Read the model definition and answer for the solid it produces. Units are mm, in the model's axes. Face numbers are marked on the shaded views. Round coordinates to 2 decimals unless told otherwise and drop trailing zeros. Order: outer loops, then holes, each group sorted by start corner. A loop starts at its lowest first (then second) coordinate and runs counter-clockwise, first axis right, second up. Notation, with made-up numbers: M 57.25,-31 L 92.25,-31 A24 ccw 92.25,-16 Z; hole C -2.75,11 d3. An arc over 180 degrees is marked long. Answer as CSV lines item,"result".
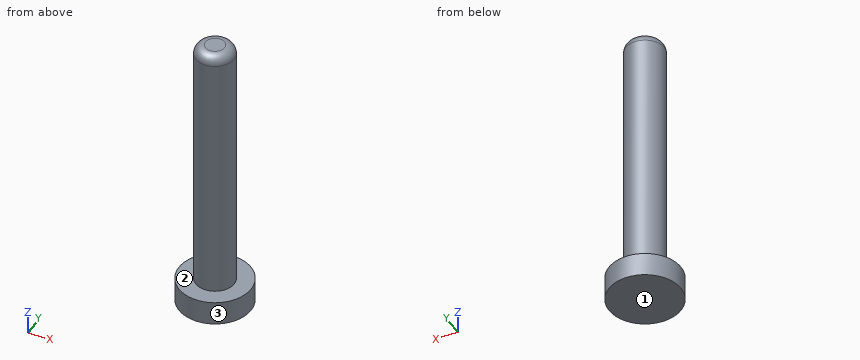
Autodesk Fusion 360 part; units mm, degrees
sketch "Skizze1" plane through (0, 0, 0) normal (0, 0, 1) x (1, 0, 0)
  circle A0 centre (0, 0) radius 7.5
  circle A1 centre (0, 0) radius 4
  dimension "d1" = 15
  dimension "d2" = 8
extrude "Extrusion1" add sketch "Skizze1" along normal blind 5
extrude "Extrusion2" add sketch "Skizze1" along normal blind 60 contours A1
fillet "Abrundung1" radius 2 1 edges at (-3.7293, -1.4465, 60)
Item 1: Flat-ended cylindrical pins translate along their axes: pin 1 (8 mm diameter, centred on x = 1, y = 4.5, fed in from +Z); pin 2 (5 mm diameter, centred on y = 4, z = 12, fed in from +X); pin 3 (5 mm diameter, centred on x = -6, z = 26, fed in from +Y); pin 4 (2 mm diameter, centred on y = 3.5, z = 25, fed in from -X). Find the tip coordinate at first contact, or state that the pin passes through.
Ans:
pin 1,"z = 60"
pin 2,"x = 3.71"
pin 3,"y = 1.94"
pin 4,"x = -3.12"
Item 2: Find the intervals of material crossed by probe 1 along Z at (x, y) = (-2.25, 5); probe 2 along X at (y, z) = (-0.25, 4.5); probe 3 along Y at (x, z) = (0, 11), in increasing order. Write a range as [from, to].
Ans:
probe 1,"[0, 5]"
probe 2,"[-7.5, 7.5]"
probe 3,"[-4, 4]"
Item 3: A cutting plane is placed at A-A, the plane x = -6. Determine the outline of the cut face in (y, z), and give its area (3 significant figures).
Ans:
outline,"M -4.5,0 L 4.5,0 L 4.5,5 L -4.5,5 Z"
area,"45.0 mm2"
Item 4: Determine the mould class of the marked faces 1, 2 and 3 for opening direction Z: +Z half, -Z half, draft (parallel to the pull), parting line (faces both ways), or undercut.
Ans:
face 1,"-Z half"
face 2,"+Z half"
face 3,"draft"
Item 5: A cutting plane is placed at B-B, the plane z = 22.5. Determine the outline of the cut face in (x, y), and give its area (3 significant figures).
Ans:
outline,"C 0,0 d8"
area,"50.3 mm2"
